Verification items for this drawing (mm, ordinates from the low corner). A direction names the side the tool comes from. Coordinates: 2 decimals unless noted, no trailing zeros. Order: outer loops, then holes, each group sorted by start corner. A loop starts at its lowest first (then second) coordinate and runs counter-clockwise, first axis right, second up. Notation, with made-up numbers: (-3, 18.5) -> (9, 18.5) arc R18 cw to (9, 53.5) -> close; hole circle Ø2 at (-21, -22). An arc over 180 degrees is marked (long way). Answer in a Markdown table with one row per item. Add a question column.
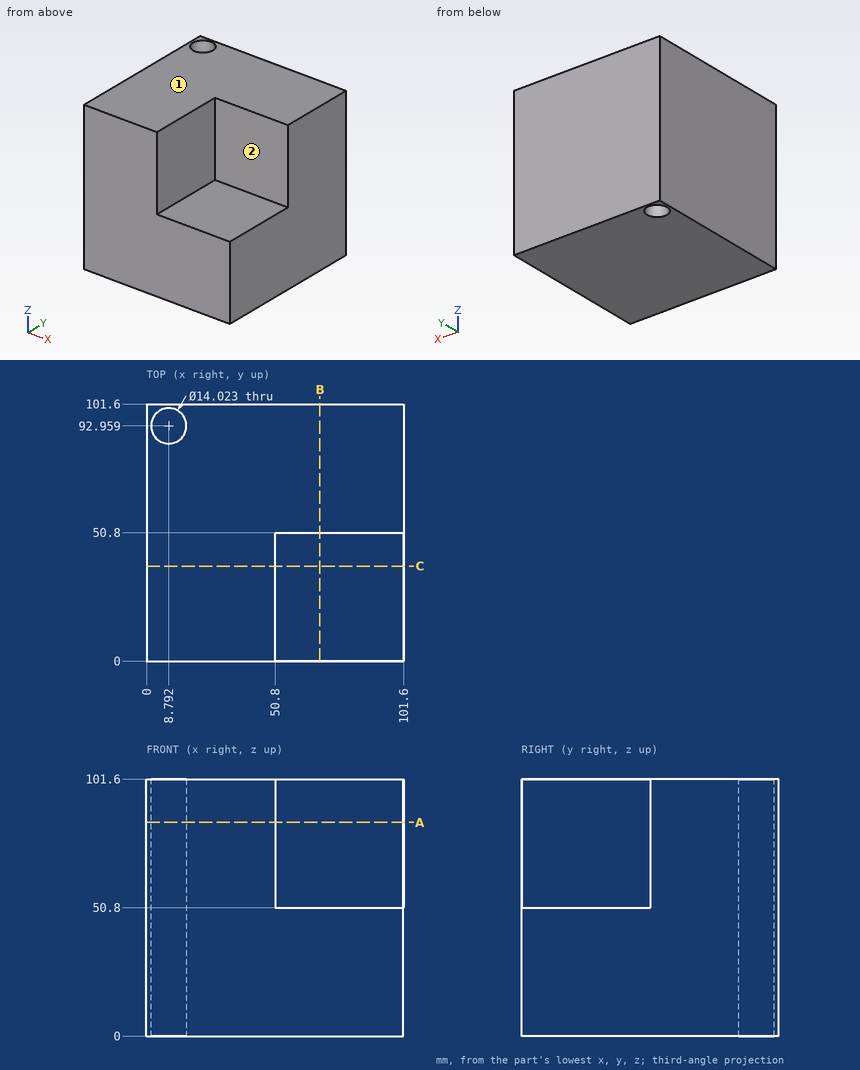
(1) Scan lines: line 1 along Y through (x, z) = (9.5, 32.5) (1 decimal); line 2 along Z through (x, y) = (82.5, 22); line 3 along X through (y, z) = (89, 82) (1 decimal). Record each from-to range of solid material in increasing order.
(2) Go/stop test with flat-tipped pins: P1, Ø12, axis at x = 87.5, y = 42.5, coming from the +Z side; P2, Ø6, axis at x = 69, z = 83.5, coming from the -Y side. Record where each tip stops, or that it passes through.
(3) Cross-section at A-A (z = 84.5). Enter the section's corners in (x, y), plus the area to 3 significant figures.
(4) Cross-section at C-C (y = 37.5). Enter the section's corners in (x, z).
(5) Cross-section at B-B (x = 68.5). Enter the section's corners in (y, z).
(6) Access from +Z, -Z, +X, -X, +Y, -Y to the whole of each face (thin tool, end or side, straight path). Record for the marked faces 1 and 2.
Checks:
| question | item | result |
|---|---|---|
| 1 | line 1 | 0 to 86, 99.9 to 101.6 |
| 1 | line 2 | 0 to 50.8 |
| 1 | line 3 | 0 to 3, 14.6 to 101.6 |
| 2 | P1 | z = 50.8 |
| 2 | P2 | y = 50.8 |
| 3 | outline | (0, 0) -> (50.8, 0) -> (50.8, 50.8) -> (101.6, 50.8) -> (101.6, 101.6) -> (0, 101.6) -> close; hole circle Ø14.02 at (8.79, 92.96) |
| 3 | area | 7,590 mm² |
| 4 | outline | (0, 0) -> (101.6, 0) -> (101.6, 50.8) -> (50.8, 50.8) -> (50.8, 101.6) -> (0, 101.6) -> close |
| 5 | outline | (0, 0) -> (101.6, 0) -> (101.6, 101.6) -> (50.8, 101.6) -> (50.8, 50.8) -> (0, 50.8) -> close |
| 6 | face 1 | +Z, +X, -X, +Y, -Y |
| 6 | face 2 | +Z, +X, -Y |
